```python
from build123d import *

# Parameters (mm, degrees)
PLAT_W                      = 30
PLAT_H                      = 5
EL_MENT_M_CANO_SOUD_1_DEPTH = 75
ENL_V_MAT_EXTRU_1_DEPTH     = 6
CONG_1_R                    = 3


with BuildPart() as part:
    # plat → Elément mécano-soudé1 (new body)
    with BuildSketch(Plane.YZ.offset(-37.5)):
        Rectangle(PLAT_W, PLAT_H)
    extrude(amount=EL_MENT_M_CANO_SOUD_1_DEPTH)

    # Esquisse2 → Enlèv. mat.-Extru.1 (cut, through all)
    with BuildSketch(Plane(origin=(0, 0, -2.5), x_dir=(-1, 0, 0), z_dir=(0, 0, -1))):
        with BuildLine():
            Line((-16.5, -15), (-10.5, -15))
            Line((-10.5, -15), (-10.5, 5))
            ThreePointArc((-10.5, 5), (-13.5, 8), (-16.5, 5))
            Line((-16.5, 5), (-16.5, -15))
        make_face()
    extrude(amount=-ENL_V_MAT_EXTRU_1_DEPTH, mode=Mode.SUBTRACT)

    # Congé1
    cong_1_edges = [part.edges().sort_by_distance(p)[0] for p in [
        (37.5, 15, 0),
        (16.5, -15, 0),
        (10.5, -15, 0),
        (37.5, -15, 0),
        (-37.5, 15, 0),
        (-37.5, -15, 0),
    ]]
    fillet(cong_1_edges, radius=CONG_1_R)


solid = part.part
```
Geometry check sheet. Reference: the model listing, model coordinates, mm. A direction names the side the tool comes from. Round coordinates to 2 decimals unless told otherwise and drop trailing zeros. Loops run counter-clockwise (first coordinate to the right, second up) from the corner with the lowest first, then second, coordinate; pieces in that order, holes last. Notation, with made-up numbers: (-36.75, 11.25) - (-18.75, 11.25) arc R29 cw to (-18.75, 44.25) - close; hole circle Ø2 at (46, 79.25). An arc over 180 degrees is marked (long way). Use a Markdown table: item, result.
Q1. Cross-section at A-A on y = -9.25. Record the cut outline in (x, z), plus the area to 3 significant figures.
Solutions:
| item | result |
|---|---|
| outline | (-37.5, -2.5) - (10.5, -2.5) - (10.5, 2.5) - (-37.5, 2.5) - close; (16.5, -2.5) - (37.5, -2.5) - (37.5, 2.5) - (16.5, 2.5) - close |
| area | 345 mm2 |
Q2. Material ranges on line 1 (X direction, y = -4.25, z = -1.2); line 2 (X direction, y = 7, z = -1.8); line 3 (X direction, y = 13.5, z = -0.7), recorded low to high.
Solutions:
| item | result |
|---|---|
| line 1 | x = -37.5 to 10.5, 16.5 to 37.5 |
| line 2 | x = -37.5 to 11.26, 15.74 to 37.5 |
| line 3 | x = -37.1 to 37.1 |
Q3. Cross-section at D-D on y = 6.5. Record the cut outline in (x, z), plus the area to 3 significant figures.
Solutions:
| item | result |
|---|---|
| outline | (-37.5, -2.5) - (10.9, -2.5) - (10.9, 2.5) - (-37.5, 2.5) - close; (16.1, -2.5) - (37.5, -2.5) - (37.5, 2.5) - (16.1, 2.5) - close |
| area | 349 mm2 |
Q4. Cross-section at B-B on z = 0.5. Record the cut outline in (x, y).
Solutions:
| item | result |
|---|---|
| outline | (-37.5, -12) arc R3 ccw to (-34.5, -15) - (7.5, -15) arc R3 ccw to (10.5, -12) - (10.5, 5) arc R3 cw to (16.5, 5) - (16.5, -12) arc R3 ccw to (19.5, -15) - (34.5, -15) arc R3 ccw to (37.5, -12) - (37.5, 12) arc R3 ccw to (34.5, 15) - (-34.5, 15) arc R3 ccw to (-37.5, 12) - close |
Q5. Go/stop test with flat-tipped pins: P1, Ø5, axis at x = 13.5, y = -4.5, coming from the +Z side; P2, Ø3, axis at x = 15.5, y = 6.5, coming from the -Z side. Record where each tip stops, or that it passes through.
Solutions:
| item | result |
|---|---|
| P1 | passes through |
| P2 | stops at z = -2.5 |
Q6. Cross-section at C-C on x = 13.5. Record the cut outline in (y, z).
Solutions:
| item | result |
|---|---|
| outline | (8, -2.5) - (15, -2.5) - (15, 2.5) - (8, 2.5) - close |
Q7. Draft check along X on faces 3 (the flat face through (10.5, -4, 0)), 4 (the cylindrical face through (-36.6, -14.14, 0.04)), 5 (the cylindrical face through (13.4, 8, 0)), 6 (the flat face through (-1, 0, -2.5)). Enter one of: released by +X, released by -X, zero draft, split by the parting line, or undercut.
Solutions:
| item | result |
|---|---|
| face 3 | undercut |
| face 4 | released by -X |
| face 5 | undercut |
| face 6 | zero draft |
Q8. Access from +Z, -Z, +X, -X, +Y, -Y to the whole of each face (thin tool, end or side, straight path). Record for faces 1 (the cylindrical face through (36.64, -14.1, 0.04)), 2 (the cylindrical face through (9.6, -14.14, 0.04)).
Solutions:
| item | result |
|---|---|
| face 1 | +Z, -Z, +X, -Y |
| face 2 | +Z, -Z, -Y |
